from build123d import *

# Parameters (mm, degrees)
SM_BASE_FLANGE_1_DEPTH           = 40
M3X0_5_1_D                       = 2.5
SKETCH_22_W                      = 3
SKETCH_22_H                      = 12
EXTRUDE_6_DEPTH                  = 29
SKETCH_23_W                      = 3
SKETCH_23_H                      = 67
EXTRUDE_7_DEPTH                  = 8
CHAMFER_1_SIZE                   = 10
CHAMFER_2_SIZE                   = 5
SM_EDGE_FLANGE_1_STRIP_CUT_DEPTH = 8
SM_EDGE_FLANGE_1_DEPTH           = 8
SM_EDGE_FLANGE_2_STRIP_CUT_DEPTH = 8
SM_EDGE_FLANGE_2_DEPTH           = 8
SM_EDGE_FLANGE_3_STRIP_CUT_DEPTH = 8
SM_EDGE_FLANGE_3_DEPTH           = 8


# Sheet-metal steps are written as plain solids
with BuildPart() as part:
    # 草圖3 → 基材-凸緣1 (new body)
    with BuildSketch(Plane.XY):
        with BuildLine():
            Line((12, 0), (1, 0))
            ThreePointArc((1, 0), (0.292893219, -0.292893219), (0, -1))
            Line((0, -1), (0, -25))
            Line((0, -25), (-3, -25))
            Line((-3, -25), (-3, -1))
            ThreePointArc((-3, -1), (-1.828427125, 1.828427125), (1, 3))
            Line((1, 3), (12, 3))
            Line((12, 3), (12, 0))
        make_face()
    extrude(amount=SM_BASE_FLANGE_1_DEPTH)

    # M3x0.5 螺紋孔1 (through all)
    with Locations(Plane(origin=(0, 3, 0), x_dir=(1, 0, 0), z_dir=(0, 1, 0))):
        with Locations((7.5, -30), (7.5, -10)):
            Hole(M3X0_5_1_D / 2)

    # 草圖22 → 填料-伸長6 (add)
    with BuildSketch(Plane.XZ.offset(25)):
        with Locations((-1.5, 34)):
            Rectangle(SKETCH_22_W, SKETCH_22_H)
    extrude(amount=EXTRUDE_6_DEPTH)

    # 草圖23 → 填料-伸長7 (add)
    with BuildSketch(Plane.XZ.offset(54)):
        with Locations((-1.5, 61.5)):
            Rectangle(SKETCH_23_W, SKETCH_23_H)
    extrude(amount=EXTRUDE_7_DEPTH)

    # 導角1
    chamfer_1_edges = [part.edges().sort_by_distance(p)[0] for p in [
        (-1.5, -54, 40),
        (-1.5, -62, 28),
    ]]
    chamfer(chamfer_1_edges, length=CHAMFER_1_SIZE)

    # 導角2
    chamfer_2_edges = [part.edges().sort_by_distance(p)[0] for p in [
        (-1.5, -25, 0),
    ]]
    chamfer(chamfer_2_edges, length=CHAMFER_2_SIZE)

    # 邊線-凸緣1 strip (across the edge) → 邊線-凸緣1 strip cut (cut)
    with BuildSketch(Plane(origin=(-3, -62, 95), x_dir=(-0.8660254037844416, 0, -0.49999999999999495), z_dir=(0, 1, 0))):
        Polygon((-9.464101615, 10.392304845), (-2.464101615, -1.732050808), (0.133974596, -0.232050808), (-6.866025404, 11.892304845), align=None)
    extrude(amount=SM_EDGE_FLANGE_1_STRIP_CUT_DEPTH, mode=Mode.SUBTRACT)

    # 邊線-凸緣1 section (across the edge) → 邊線-凸緣1 (add)
    with BuildSketch(Plane(origin=(-3, -62, 95), x_dir=(-0.8660254037844416, 0, -0.49999999999999495), z_dir=(0, 1, 0))):
        with BuildLine():
            Line((-3, 0.267949192), (-3, 45))
            Line((-3, 45), (0, 45))
            Line((0, 45), (0, 0.267949192))
            ThreePointArc((0, 0.267949192), (0.034074174, 0.009130147), (0.133974596, -0.232050808))
            Line((0.133974596, -0.232050808), (-2.464101615, -1.732050808))
            ThreePointArc((-2.464101615, -1.732050808), (-2.863703305, -0.767326988), (-3, 0.267949192))
        make_face()
    extrude(amount=SM_EDGE_FLANGE_1_DEPTH)

    # 邊線-凸緣2 strip (across the edge) → 邊線-凸緣2 strip cut (cut)
    with BuildSketch(Plane(origin=(-25.5, -62, 133.97114317), x_dir=(0, 0, -1), z_dir=(0, 1, 0))):
        Polygon((-13.124355653, 4.113248654), (-1, -2.886751346), (0.5, -0.288675135), (-11.624355653, 6.711324865), align=None)
    extrude(amount=SM_EDGE_FLANGE_2_STRIP_CUT_DEPTH, mode=Mode.SUBTRACT)

    # 邊線-凸緣2 section (across the edge) → 邊線-凸緣2 (add)
    with BuildSketch(Plane(origin=(-25.5, -62, 133.97114317), x_dir=(0, 0, -1), z_dir=(0, 1, 0))):
        with BuildLine():
            Line((-3, 0.577350269), (-3, 50))
            Line((-3, 50), (0, 50))
            Line((0, 50), (0, 0.577350269))
            ThreePointArc((0, 0.577350269), (0.133974596, 0.077350269), (0.5, -0.288675135))
            Line((0.5, -0.288675135), (-1, -2.886751346))
            ThreePointArc((-1, -2.886751346), (-2.464101615, -1.422649731), (-3, 0.577350269))
        make_face()
    extrude(amount=SM_EDGE_FLANGE_2_DEPTH)

    # 邊線-凸緣3 strip (across the edge) → 邊線-凸緣3 strip cut (cut)
    with BuildSketch(Plane(origin=(-75.5, -62, 133.97114317), x_dir=(0.8660254037844312, 0, -0.5000000000000132), z_dir=(0, 1, 0))):
        Polygon((-13.124355653, 4.113248654), (-1, -2.886751346), (0.5, -0.288675135), (-11.624355653, 6.711324865), align=None)
    extrude(amount=SM_EDGE_FLANGE_3_STRIP_CUT_DEPTH, mode=Mode.SUBTRACT)

    # 邊線-凸緣3 section (across the edge) → 邊線-凸緣3 (add)
    with BuildSketch(Plane(origin=(-75.5, -62, 133.97114317), x_dir=(0.8660254037844312, 0, -0.5000000000000132), z_dir=(0, 1, 0))):
        with BuildLine():
            Line((-3, 0.577350269), (-3, 45))
            Line((-3, 45), (0, 45))
            Line((0, 45), (0, 0.577350269))
            ThreePointArc((0, 0.577350269), (0.133974596, 0.077350269), (0.5, -0.288675135))
            Line((0.5, -0.288675135), (-1, -2.886751346))
            ThreePointArc((-1, -2.886751346), (-2.464101615, -1.422649731), (-3, 0.577350269))
        make_face()
    extrude(amount=SM_EDGE_FLANGE_3_DEPTH)


solid = part.part
For this review, take the finished solid that the model builds, in its own axes (mm). A direction names the side the tool comes from. Coordinates: 2 decimals unless noted, no trailing zeros. Order: outer loops, then holes, each group sorted by start corner. A loop starts at its lowest first (then second) coordinate and runs counter-clockwise, first axis right, second up. Notation, with made-up numbers: (-19, 0) - (10, 0) arc R17 cw to (10, 32) - close; hole circle Ø10 at (0, 10.5). An arc over 180 degrees is marked (long way). Answer as CSV lines item,"result". Start each with the question number.
1) Add section A-A (z = 35.5). State the section outline as (x, y) points, then the cut area to 3 significant figures.
2) To check wall thickness, follow line 1 along Z through (x, y) = (7.5, 1.45); line 2 along Z through (x, y) = (7, 1); line 3 along X through (y, z) = (1, 30). State the ranges of each line that lie inside material, in increasing order. Write a range as [from, to].
3) Add section D-D (x = -58). State the section outline as (y, z) points, then the cut area to 3 significant figures.
4) Machinability: for faces 4 (the flat face through (-89.34, -58.06, 116)), 5 (the flat face through (-14.327, -58.056, 114.619)), 6 (the flat face through (7, 0, 20)), 7 (the flat face through (-1, -25, 16)), 8 (the flat face through (-1, -15, 40)), which of the approach directions +Z, -Z, +X, -X, +Y, -Y give a long, thin tool a straight path to every point of the face, cutting with its end or side? Answer none if there is none.
5) Insertion check: P1, Ø7.5, axis at x = 1.5, y = -11.5, coming from the +Z side; P2, Ø1.5, axis at x = -1.5, z = 13, coming from the -Y side; P3, Ø6, axis at y = -51, z = 37, coming from the -X side. Each pin has a flat end and moves straight along its axis. Give the tip position at first contact, or say it passes through.
6) Add section B-B (y = -30.5). State the section outline as (x, z) points, then the cut area to 3 significant figures.
7) Draft analysis for pull direction X (two halves, no side actions). For faces 1 (the cylindrical face through (-1.859, 1.797, 19.72)), 2 (the flat face through (-87.05, -58.056, 113.966)), 3 (the flat face through (-11.42, -58.06, 115.58)), state which applies: +X half, -X half, draft (parallel to the pull), parting line (faces both ways), or undercut.
8) Add section C-C (z = 118). State the section outline as (x, y) points.
Result:
1,outline,"(-3, -59.5) - (0, -59.5) - (0, -1) arc R1 cw to (1, 0) - (12, 0) - (12, 3) - (1, 3) arc R4 ccw to (-3, -1) - close"
1,area,"220 mm^2"
2,line 1,"[0, 8.75], [11.25, 28.75], [31.25, 40]"
2,line 2,"[0, 8.85], [11.15, 28.85], [31.15, 40]"
2,line 3,"[-2.46, 6.25], [8.75, 12]"
3,outline,"(-62, 133.97) - (-54, 133.97) - (-54, 136.97) - (-62, 136.97) - close"
3,area,"24.0 mm^2"
4,face 4,"+Z, -X, +Y, -Y"
4,face 5,"-Z, +Y, -Y"
4,face 6,"+Z, -Z, +X, -Y"
4,face 7,"-Z, +X, -X, -Y"
4,face 8,"+Z, +X, -X, +Y"
5,P1,"z = 40"
5,P2,"y = -25"
5,P3,"x = -3"
6,outline,"(-3, 28) - (0, 28) - (0, 40) - (-3, 40) - close"
6,area,"36.0 mm^2"
7,face 1,"-X half"
7,face 2,"undercut"
7,face 3,"+X half"
8,outline,"(-88.19, -62) - (-84.72, -62) - (-84.72, -54) - (-88.19, -54) - close; (-16.28, -62) - (-12.81, -62) - (-12.81, -54) - (-16.28, -54) - close"
